The drawing under review shows one solid part. Ordinate dimensions are in mm from its lowest x, y, z. A direction names the side the tool comes from. Give positions to 0.01 mm unless a question says otherwise; leave off trailing zeros. Write each loop counter-clockwise with the first axis right and the second up, starting at its lowest first coordinate (ties: lowest second). Pieces come first, ordered by that corner, then holes. Notation, with made-up numbers: M 84.5,25 L 107.5,25 A16 cw 107.5,37 Z; hole C -16.5,-30 d5. An arc over 180 degrees is marked long. Write item = value, one per line. Start each with the question number.
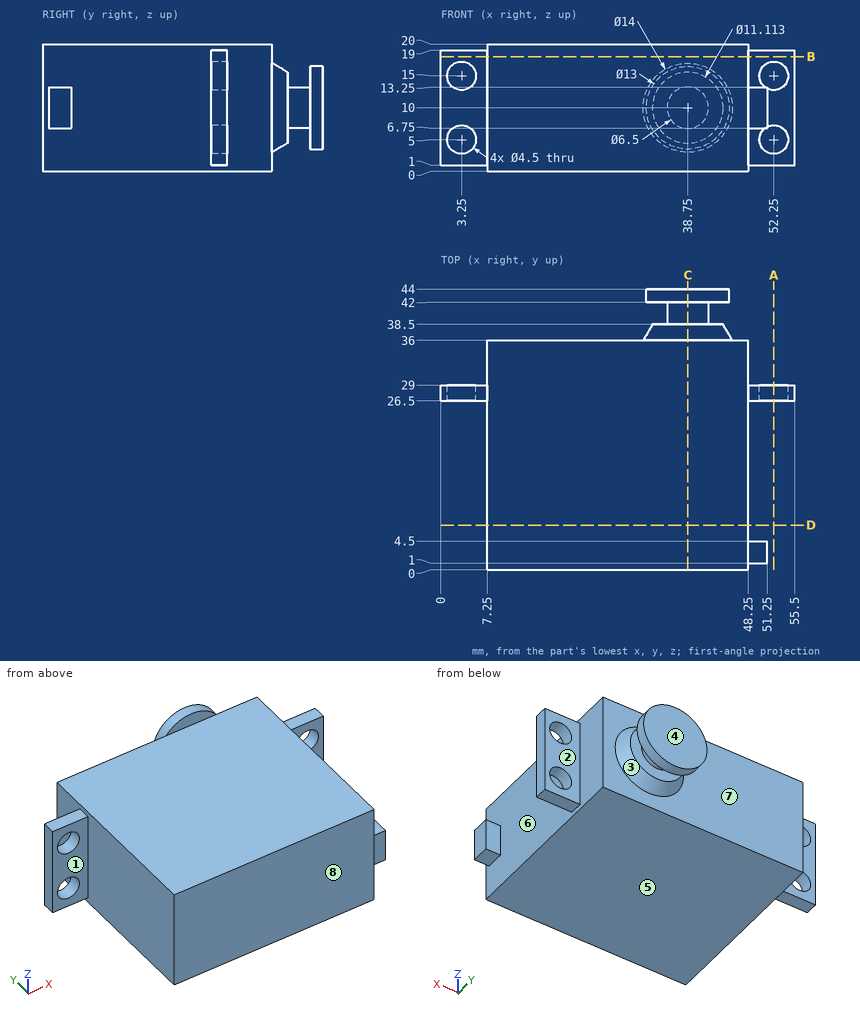
Item 1: The part is to be moulded in two halves that separate along Y. For the marked faces 6, 7 and 8, say which applies: released by +Y, released by -Y, zero draft, split by the parting line, or undercut.
Item 2: We need section B-B, the plane z = 18. Write out the cut boundary in (x, y), and give its area (3 significant figures).
Item 3: Clearance check with flat-ended pins moving along their axes: P1, Ø3.5, axis at x = 52.25, z = 15, coming from the +Y side; P2, Ø0.8, axis at x = 4, y = 28, coming from the +Z side; P3, Ø5, axis at y = 10, z = 12.5, coming from the +X side; P4, Ø3.5, axis at x = 52, z = 7.5, coming from the +Y side. State where each tip first meets the part, or that it passes through.
Item 4: We need section A-A, the plane x = 52.25. Write out the cut boundary in (y, z), and give its area (3 significant figures).
Item 5: For the marked faces 1, 2, 3, 4 and 5, list the 3-axis set-ups (+Z, -Z, +X, -X, +Y, -Y) from which the entire face can be reached by the end or side of a thin tool; tool diameter is ignored.
Item 6: We need section D-D, the plane y = 7. Write out the cut boundary in (x, z), and give its area (3 significant figures).
Item 7: We need section C-C, the plane x = 38.75. Write out the cut boundary in (y, z).
Item 8: To check wall thickness, follow probe 1 along Z at (x, y) = (52, 27); probe 2 along X at (y, z) = (27.4, 15); probe 3 along X at (y, z) = (5.5, 9). State the ranges of each line that lie inside material, in increasing order. Write a range as [from, to].
Worked out:
q1.face_6 = undercut
q1.face_7 = released by +Y
q1.face_8 = released by -Y
q2.outline = M 0,26.5 L 7.25,26.5 L 7.25,0 L 48.25,0 L 48.25,26.5 L 55.5,26.5 L 55.5,29 L 48.25,29 L 48.25,36 L 7.25,36 L 7.25,29 L 0,29 Z
q2.area = 1,510 mm²
q3.P1 = through
q3.P2 = 19
q3.P3 = 48.25
q3.P4 = 29
q4.outline = M 26.5,1 L 29,1 L 29,2.75 L 26.5,2.75 Z; M 26.5,7.25 L 29,7.25 L 29,12.75 L 26.5,12.75 Z; M 26.5,17.25 L 29,17.25 L 29,19 L 26.5,19 Z
q4.area = 22.5 mm²
q5.face_1 = +Z, -Z, -X, -Y
q5.face_2 = +Z, -Z, +X, +Y
q5.face_3 = none
q5.face_4 = +Z, -Z, +X, -X, +Y
q5.face_5 = -Z, +X, -X, +Y, -Y
q6.outline = M 7.25,0 L 48.25,0 L 48.25,20 L 7.25,20 Z
q6.area = 820 mm²
q7.outline = M 0,0 L 36,0 L 36,3 L 38.5,4.44 L 38.5,6.75 L 42,6.75 L 42,3.5 L 44,3.5 L 44,16.5 L 42,16.5 L 42,13.25 L 38.5,13.25 L 38.5,15.56 L 36,17 L 36,20 L 0,20 Z
q8.probe_1 = [1, 2.76], [7.24, 12.76], [17.24, 19]
q8.probe_2 = [0, 1], [5.5, 50], [54.5, 55.5]
q8.probe_3 = [7.25, 48.25]
